Drawing for the job (mm, zero at the part's lowest x, y, z). A direction names the side the tool comes from. Give positions to 0.01 mm unless a question says otherwise; leave off trailing zeros. Order: outer loops, then holes, each group sorted by start corner. A loop starts at its lowest first (then second) coordinate and runs counter-clockwise, first axis right, second up. Notation, with made-up numbers: (46, 41.5) - (50, 41.5) arc R30 cw to (50, 65.5) - close; hole circle Ø1 at (43, 74). An arc over 180 degrees is marked (long way). Use a Markdown table: item, result. Add a question column.
(1) Slice it at A-A (z = 42). Write the cut outline in (x, y), then the cut area to 3 significant figures.
(2) Mould opens along Y. For the marked faces 3, 4, 5 and 6 say: +Y half, -Y half, draft (parallel to the pull), parting line (faces both ways), or undercut.
(3) Slice it at C-C (x = 51.5). Write the cut outline in (y, z).
(4) Flat gauge pin, fed straight in: pin 1 (8 mm diameter, centred on x = 66, y = 34, fed in from +Z). Where does the tip first touch, or does it go through?
(5) Slice it at B-B (y = 65). Write the cut outline in (x, z).
(6) Which spindle directions (+Z, -Z, +X, -X, +Y, -Y) get a long thin tool onto all of the face, cutting with end or side? Do the marked faces 1 and 2. Say none if no direction does.
(7) Wall check: line 1 (X direction, y = 96.5, z = 6); line 2 (Y direction, x = 69.5, z = 17.5); line 3 (Z direction, x = 12, y = 73). Give the ranges that are in metal, low to high.
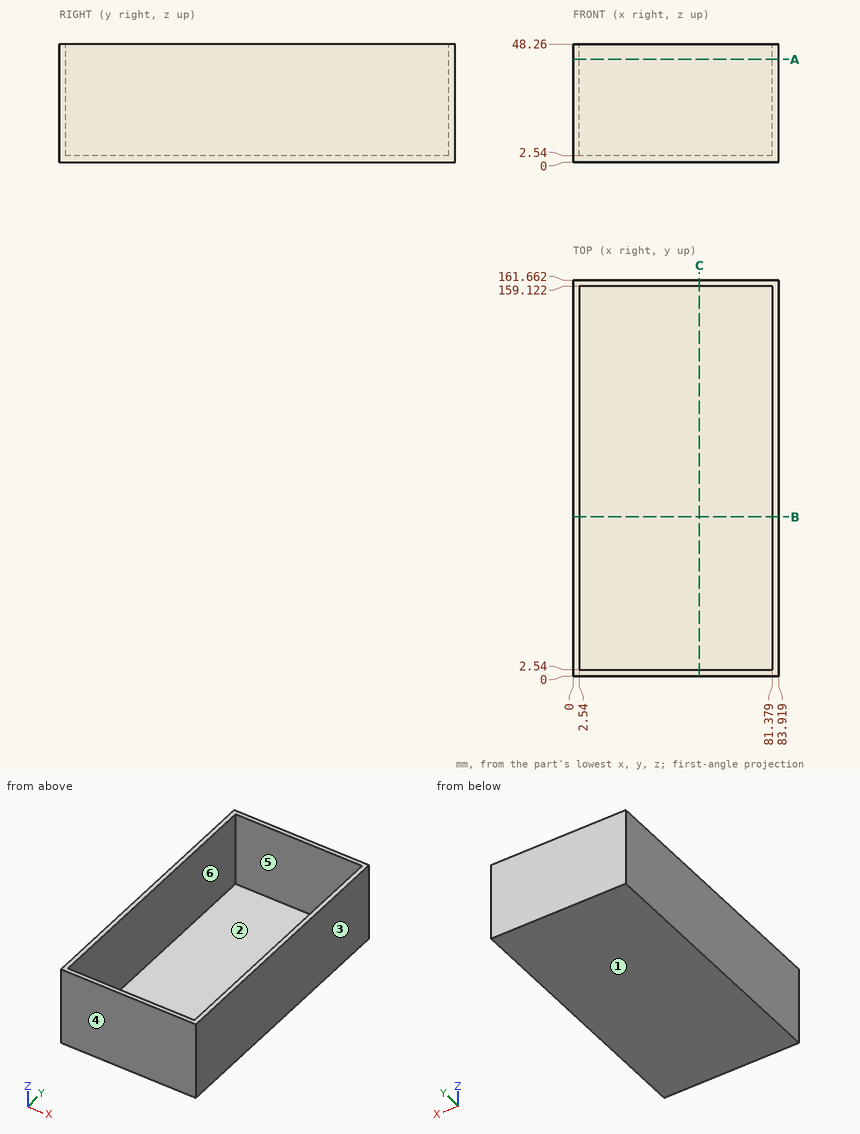
Solution:
| question | item | result |
|---|---|---|
| 1 | outline | (0, 0) - (83.92, 0) - (83.92, 161.66) - (0, 161.66) - close; hole (2.54, 2.54) - (81.38, 2.54) - (81.38, 159.12) - (2.54, 159.12) - close |
| 1 | area | 1,220 mm2 |
| 2 | face 3 | draft |
| 2 | face 4 | -Y half |
| 2 | face 5 | undercut |
| 2 | face 6 | undercut |
| 3 | outline | (0, 0) - (161.66, 0) - (161.66, 48.26) - (159.12, 48.26) - (159.12, 2.54) - (2.54, 2.54) - (2.54, 48.26) - (0, 48.26) - close |
| 4 | pin 1 | z = 2.54 |
| 5 | outline | (0, 0) - (83.92, 0) - (83.92, 48.26) - (81.38, 48.26) - (81.38, 2.54) - (2.54, 2.54) - (2.54, 48.26) - (0, 48.26) - close |
| 6 | face 1 | -Z, +X, -X, +Y, -Y |
| 6 | face 2 | +Z |
| 7 | line 1 | 0 to 2.54, 81.38 to 83.92 |
| 7 | line 2 | 0 to 2.54, 159.12 to 161.66 |
| 7 | line 3 | 0 to 2.54 |
